Geometry: see drawing. Coordinates: mm, zero at the bounding-box minimum. A direction names the side the tool comes from. Coordinates: 2 decimals unless noted, no trailing zeros. Write each loop counter-clockwise with the first axis right and the second up, starting at its lowest first coordinate (ties: lowest second). Pieces come first, ordered by that corner, then holes.
1) Section query A-A (z = 3.25). Output: boundary loops of the cut face in (x, y).
2) Set-up query: the marked faces 1 and 2. Return all of +Z, -Z, +X, -X, +Y, -Y with unobstructed straight access to the full face (end or side cutting, diameter ignored); none if empty.
3) Draft query along X for the marked faces 3, 4 and 5. Return one class per face: pulls with the +X half, pulls with the -X half, needs draft (parallel to the pull), parting line crosses it, or undercut.
4) Section query B-B (z = 11.25). Output: boundary loops of the cut face in (x, y).
5) Section query D-D (x = 0.95). Output: boundary loops of the cut face in (y, z) (1 decimal), then the cut area to 3 significant figures.
6) Pin query (flat end, axial travel): pin 1 Ø1.5 at (x, y) = (2, 1.5) entering from +Z. Return the tip coordinate at first contact, or that it passes through.
7) Line query: L1, parallel to X at y = 2.95, z = 6 (1 decimal); L2, parallel to Z at x = 1.85, y = 0.75; L3, parallel to Y at x = 2.5, z = 14. Output: solid intervals per line, ascending.
8) Section query C-C (y = 4.95). Output: boundary loops of the cut face in (x, z), then the cut area to 3 significant figures.
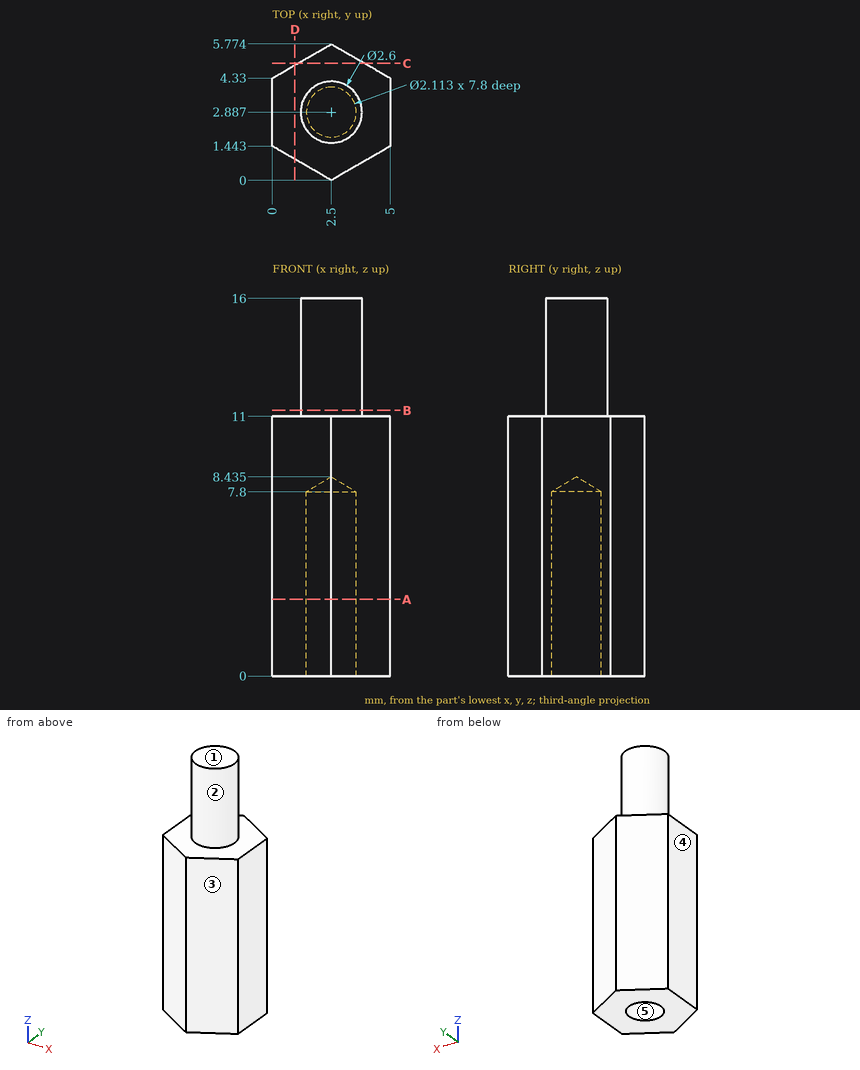
Answer:
1. outline: (0, 1.44) - (2.5, 0) - (5, 1.44) - (5, 4.33) - (2.5, 5.77) - (0, 4.33) - close; hole circle Ø2.11 at (2.5, 2.89)
2. face 1: +Z, +X, -X, +Y, -Y
2. face 2: +Z
3. face 3: pulls with the +X half
3. face 4: pulls with the -X half
3. face 5: undercut
4. outline: circle Ø2.6 at (2.5, 2.89)
5. outline: (0.9, 0) - (4.9, 0) - (4.9, 11) - (0.9, 11) - close
5. area: 43.8 mm2
6. pin 1: stops at z = 16
7. L1: x = 0 to 1.4, 3.6 to 5
7. L2: z = 0 to 11
7. L3: y = 1.59 to 4.19
8. outline: (1.07, 0) - (3.93, 0) - (3.93, 11) - (1.07, 11) - close
8. area: 31.4 mm2
